```python
from build123d import *

# Parameters (mm, degrees)
F0_R     = 4.15
F1_DEPTH = 10
F2_R     = 1.65
F3_DEPTH = 25


with BuildPart() as f1:
    # F0 (on Top) → F1 (new body)
    with BuildSketch(Plane.XY):
        with BuildLine():
            Line((6.873864, -5), (6.873864, 5))
            ThreePointArc((6.873864, 5), (-8.5, 0), (6.873864, -5))
        make_face()
        Circle(F0_R, mode=Mode.SUBTRACT)
        with BuildLine():
            ThreePointArc((6.873864, -5), (8.083249, -2.628893), (8.5, 0))
            ThreePointArc((8.5, 0), (8.083249, 2.628893), (6.873864, 5))
            Line((6.873864, 5), (6.873864, -5))
        make_face()
        with BuildLine():
            ThreePointArc((6.873864, 5), (8.083249, 2.628893), (8.5, 0))
            ThreePointArc((8.5, 0), (8.083249, -2.628893), (6.873864, -5))
            Line((6.873864, -5), (36.873864, -5))
            Line((36.873864, -5), (36.873864, 5))
            Line((36.873864, 5), (6.873864, 5))
        make_face()
    extrude(amount=F1_DEPTH)

    # F2 (on face) → F3 (cut)
    with BuildSketch(Plane.XZ.offset(5)):
        with Locations((11.873864, 5)):
            Circle(F2_R)
        with Locations((16.873864, 5)):
            Circle(F2_R)
        with Locations((21.873864, 5)):
            Circle(F2_R)
        with Locations((26.873864, 5)):
            Circle(F2_R)
        with Locations((31.873864, 5)):
            Circle(F2_R)
    extrude(amount=-F3_DEPTH, mode=Mode.SUBTRACT)


solid = f1.part
```
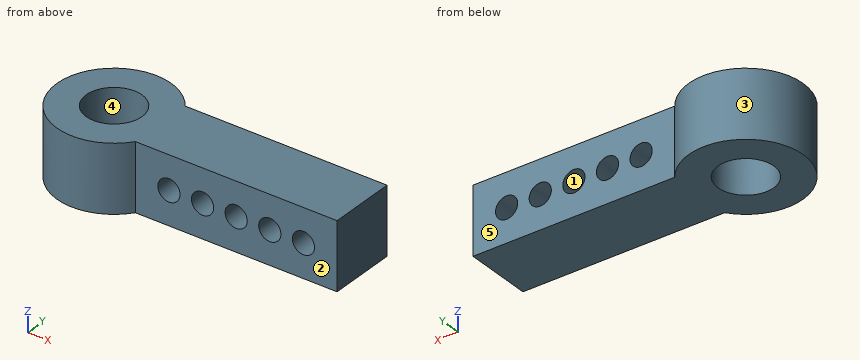
CAD build for the part. Positions are in the model's coordinates, mm. Face numbers are marked on the shaded views. A direction names the side the tool comes from. Coordinates: 2 decimals unless noted, no trailing zeros. Order: outer loops, then holes, each group sorted by start corner. A loop starts at its lowest first (then second) coordinate and runs counter-clockwise, first axis right, second up.
(1) Saw through at D-D, the plane z = 2.75. Write the cut outline in (x, y), and give its area (3 significant figures).
Solution:
outline: (6.87, -5) - (36.87, -5) - (36.87, 5) - (6.87, 5) arc R8.5 ccw (long way) to start; hole circle Ø8.3 at (0, 0)
area: 462 mm2
(2) Saw through at C-C, the plane x = 0. Write the cut outline in (y, z), and give its area (3 significant figures).
Solution:
outline: (-8.5, 0) - (-4.15, 0) - (-4.15, 10) - (-8.5, 10) - close; (4.15, 0) - (8.5, 0) - (8.5, 10) - (4.15, 10) - close
area: 87.0 mm2
(3) Saw through at A-A, the plane z = 5. Write the cut outline in (x, y).
Solution:
outline: (6.87, -5) - (10.22, -5) - (10.22, 5) - (6.87, 5) arc R8.5 ccw (long way) to start; (13.52, -5) - (15.22, -5) - (15.22, 5) - (13.52, 5) - close; (18.52, -5) - (20.22, -5) - (20.22, 5) - (18.52, 5) - close; (23.52, -5) - (25.22, -5) - (25.22, 5) - (23.52, 5) - close; (28.52, -5) - (30.22, -5) - (30.22, 5) - (28.52, 5) - close; (33.52, -5) - (36.87, -5) - (36.87, 5) - (33.52, 5) - close; hole circle Ø8.3 at (0, 0)
(4) Mould opens along X. For the marked faces 3, 4 and 5 say: released by +X, released by -X, zero draft, split by the parting line, or undercut.
Solution:
face 3: split by the parting line
face 4: undercut
face 5: zero draft
(5) Which spindle directions (+Z, -Z, +X, -X, +Y, -Y) get a long thin tool onto all of the face, cutting with end or side? Do the marked faces 1 and 2. Say none if no direction does.
Solution:
face 1: +Y, -Y
face 2: +Z, -Z, +X, -Y
(6) Drill centre lines: L1, parallel to X at y = -2.75, z = 8.5; L2, parallel to X at y = 1.5, z = 7.5; L3, parallel to Y at x = 2.5, z = 3.5. Where is each one in solid material? Low to high.
Solution:
L1: x = -8.04 to -3.11, 3.11 to 36.87
L2: x = -8.37 to -3.87, 3.87 to 36.87
L3: y = -8.12 to -3.31, 3.31 to 8.12
(7) Saw through at B-B, the plane y = 0. Write the cut outline in (x, z), and give its area (3 significant figures).
Solution:
outline: (-8.5, 0) - (-4.15, 0) - (-4.15, 10) - (-8.5, 10) - close; (4.15, 0) - (36.87, 0) - (36.87, 10) - (4.15, 10) - close; hole circle Ø3.3 at (11.87, 5); hole circle Ø3.3 at (16.87, 5); hole circle Ø3.3 at (21.87, 5); hole circle Ø3.3 at (26.87, 5); hole circle Ø3.3 at (31.87, 5)
area: 328 mm2
(8) Pin check, flat tips, straight feed: pin 1 Ø5 at (x, z) = (22, 6.5) entering from +Y; pin 2 Ø4.5 at (x, z) = (21.87, 5) entering from -Y; pin 3 Ø4 at (y, z) = (-3, 1) entering from -X; pin 4 Ø3 at (x, z) = (26.87, 5) entering from +Y. Stop position of each tip, or through.
Solution:
pin 1: stops at y = 5
pin 2: stops at y = -5
pin 3: stops at x = -8.44
pin 4: passes through
